Input: part model. Units: mm. Frame: model coordinates. Face numbers are marked on the shaded views. A direction names the side the tool comes from. Round coordinates to 2 decimals unless told otherwise and drop trailing zeros. Write each loop counter-clockwise with the first axis right and the second up, starting at its lowest first coordinate (ties: lowest second). Pieces come first, ordered by that corner, then holes. Notation, with made-up numbers: (10.5, -6) -> (17.5, -6) arc R21 ccw to (17.5, 25) -> close; hole circle Ø10 at (86.25, 49). An arc over 180 degrees is marked (long way). Write item = value, one per line.
Autodesk Inventor part; units mm, degrees
ref_plane "Work Plane1" through (1.525, 0, 0) normal (0, 0, 1) x (1, 0, 0)
ref_plane "YZ Plane" through (0, 0, 0) normal (1, 0, 0) x (0, 1, 0)
ref_plane "XZ Plane" through (0, 0, 0) normal (0, 1, 0) x (-1, 0, 0)
sketch "Sketch1" plane through (0, 0, 0) normal (0, 0, 1) x (1, 0, 0)
  line L0 (0, 12) -> (120, 12)
  line L1 (120, 12) -> (120, 0)
  line L2 (120, 0) -> (0, 0)
  line L3 (-24, 0) -> (144, 0)
  line L4 (0, -2.4) -> (0, 14.4)
  line L5 (0, 12) -> (0, 0)
  dimension "d2" = 24
  dimension "d59" = 120
revolve "Body" add sketch "Sketch1" angle 360 about axis through (120, 0, 0) along (-1, 0, 0)
sketch "Sketch2" plane through (0, 0, 0) normal (-1, 0, 0) x (0, 0, 1)
  line L0 (0, 20.7846) -> (18, 10.3923)
  line L1 (18, 10.3923) -> (18, -10.3923)
  line L2 (18, -10.3923) -> (0, -20.7846)
  line L3 (0, -20.7846) -> (-18, -10.3923)
  line L4 (-18, -10.3923) -> (-18, 10.3923)
  line L5 (-18, 10.3923) -> (0, 20.7846)
  line L6 (-25.2, 0) -> (25.2, 0)
  line L7 (0, 29.0985) -> (0, -29.0985)
  point P0 (0, 0)
  point P1 (0, 0)
  dimension "d11" = 36
extrude "Head" add sketch "Sketch2" along normal blind 15.9
sketch "Sketch4" plane through (0, 0, 0) normal (0, 0, 1) x (1, 0, 0)
  line L0 (-13.8215, 21.6) -> (-15.9, 18)
  line L1 (-1.1, 0) -> (-0.234, 0)
  line L2 (-19.0332, 0) -> (2.8992, 0)
  line L3 (-15.9, 21.6) -> (-13.8215, 21.6)
  line L4 (-15.9, 18) -> (-15.9, 21.6)
  line L5 (0, 25.92) -> (0, -4.32)
  dimension "d65" = 36
  dimension "d67" = 30
  dimension "d68" = 43.2
  dimension "d69" = 15.9
revolve "Chamfer1" cut sketch "Sketch4" angle 360 about axis through (-1.1, 0, 0) along (1, 0, 0)
thread "Thread"
chamfer "Chamfer2" distance 1.8403 distance2 1.8405 1 edges at (120, -12, 0) measured on face at (120, -3.5418, -1.8589)
fillet "Fillet" radius 0.8 1 edges at (0, -12, 0)
ref_plane "Work Plane1" through (1.525, 0, 0) normal (0, 0, 1) x (1, 0, 0)
equation "\"d2\" = GD"
equation "\"d59\" = NLG"
equation "\"d11\" = SW"
equation "\"d3\" = KOH"
equation "\"d15\" = GEL"
equation "\"d6\" = -0.5 * SPD + 0.5 * GD"
equation "\"d71\" = RR1"
equation "\"d65\" = SW"
equation "\"d67\" = ANG1"
equation "\"d68\" = 1.2 * SW"
equation "\"d69\" = KOH"
equation "\"NLG\" = 120"
equation "\"GD\" = NND"
equation "\"BDM\" = NND"
equation "\"KOH\" = 15.9"
equation "\"GEL\" = 54"
equation "\"SW\" = 36"
equation "\"SW0\" = SW"
equation "\"SPD\" = NND - 1.2269 * PTC"
equation "\"SD2\" = NND"
equation "\"SD\" = 0"
equation "\"ANG1\" = 30deg"
equation "\"GAL\" = 0.61345 * PTC"
equation "\"GUL\" = 0.61345 * PTC"
equation "\"RR\" = 0.1"
equation "\"RR1\" = 0.8"
equation "\"GD1\" = THREADDIA - 1.2269 * PTC"
equation "\"THREADDIA\" = 24"
equation "\"TOA\" = 30deg"
equation "\"PTC\" = 3"
equation "\"KOH1\" = 10.5"
equation "\"NND\" = 24"
equation "\"E0\" = 1.155 * SW"
properties part number "ANSI B18.2.3.5M - M24 x 3 x 120" material "Steel, Mild"
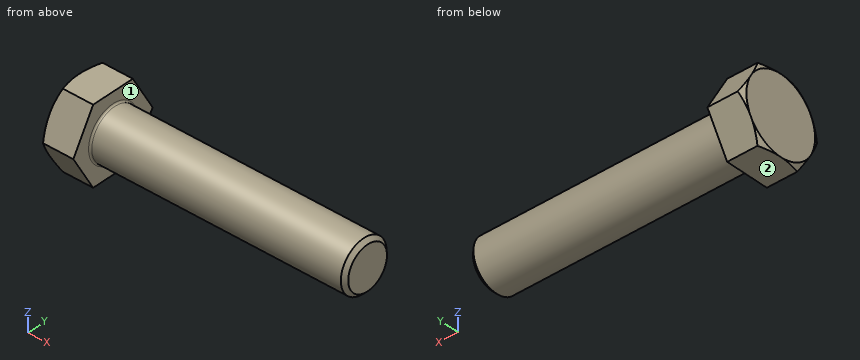
1) Line query: L1, parallel to X at y = -16.5, z = -5.5; L2, parallel to Y at x = 72, z = 0; L3, parallel to Z at x = 86, y = 11. Output: solid intervals per line, ascending. Write a range as from..to.
Solutions:
L1 = -15.9..0
L2 = -12..12
L3 = -4.8..4.8
2) Cut plane A-A (x = 72). Return the cut outline in (y, z), and give its area (3 significant figures).
Solutions:
outline = circle Ø24 at (0, 0)
area = 452 mm^2
3) Access query for the marked faces 1 and 2. Directions: +Z, -Z, +X, -X, +Y, -Y. A direction counts if a zero-diameter tool reaches every point of the face in a straight line with its end or side. Return the directions, or none.
Solutions:
face_1 = +X
face_2 = -Z, +X, -X, +Y, -Y
4) First-contact query: P1, Ø10, axis at x = 35.5, z = 0, coming from the +Y side; P2, Ø4, axis at x = 31, z = 1.5, coming from the -Y side; P3, Ø8, axis at x = 41, z = 8, coming from the +Y side. Flat tips, straight axial feed; report the tip coordinate or a pass-through.
Solutions:
P1 = 12
P2 = -12
P3 = 11.31
